Check sheet for the modelled part. Datum: model origin and axes. Units: mm. Face numbers are marked on the shaded views. A direction names the side the tool comes from. Round coordinates to 2 decimals unless told otherwise and drop trailing zeros. Write each loop counter-clockwise with the first axis right and the second up, starting at its lowest first coordinate (ties: lowest second). Pieces come first, ordered by that corner, then holes. Notation, with made-up numbers: M 16.5,60.5 L 57.5,60.5 A22 ccw 57.5,74.5 Z; hole C -37,60.25 d2. An arc over 180 degrees is marked long. Answer in a Markdown table with one row per item.
```python
from build123d import *

# Parameters (mm, degrees)
F0_R     = 11
F1_DEPTH = 1
F2_R     = 9
F3_DEPTH = 7
F4_R     = 11
F5_DEPTH = 8
F6_R     = 0.6
F7_DEPTH = 7
F8_R     = 2.5
F9_DEPTH = 16.001
F10_SIZE = 0.25


with BuildPart() as f1:
    # F0 (on Front) → F1 (new body)
    with BuildSketch(Plane.XZ):
        Circle(F0_R)
    extrude(amount=F1_DEPTH)

    # F2 (on face) → F3 (join)
    with BuildSketch(Plane.XZ.offset(1)):
        Circle(F2_R)
    extrude(amount=F3_DEPTH)

    # F4 (on face) → F5 (join)
    with BuildSketch(Plane.XZ.offset(8)):
        Circle(F4_R)
    extrude(amount=F5_DEPTH)

    # F6 (on face) → F7 (cut, through all)
    with BuildSketch(Plane.XZ.offset(1)):
        with Locations((0, 9)):
            Circle(F6_R)
        with Locations((-1.871205, 8.803328)):
            Circle(F6_R)
        with Locations((-3.66063, 8.221909)):
            Circle(F6_R)
        with Locations((-5.290067, 7.281153)):
            Circle(F6_R)
        with Locations((-6.688303, 6.022175)):
            Circle(F6_R)
        with Locations((-7.794229, 4.5)):
            Circle(F6_R)
        with Locations((-8.559509, 2.781153)):
            Circle(F6_R)
        with Locations((-8.950697, 0.940756)):
            Circle(F6_R)
        with Locations((-8.950697, -0.940756)):
            Circle(F6_R)
        with Locations((-8.559509, -2.781153)):
            Circle(F6_R)
        with Locations((-7.794229, -4.5)):
            Circle(F6_R)
        with Locations((-6.688303, -6.022175)):
            Circle(F6_R)
        with Locations((-5.290067, -7.281153)):
            Circle(F6_R)
        with Locations((-3.66063, -8.221909)):
            Circle(F6_R)
        with Locations((-1.871205, -8.803328)):
            Circle(F6_R)
        with Locations((0, -9)):
            Circle(F6_R)
        with Locations((1.871205, -8.803328)):
            Circle(F6_R)
        with Locations((3.66063, -8.221909)):
            Circle(F6_R)
        with Locations((5.290067, -7.281153)):
            Circle(F6_R)
        with Locations((6.688303, -6.022175)):
            Circle(F6_R)
        with Locations((7.794229, -4.5)):
            Circle(F6_R)
        with Locations((8.559509, -2.781153)):
            Circle(F6_R)
        with Locations((8.950697, -0.940756)):
            Circle(F6_R)
        with Locations((8.950697, 0.940756)):
            Circle(F6_R)
        with Locations((8.559509, 2.781153)):
            Circle(F6_R)
        with Locations((7.794229, 4.5)):
            Circle(F6_R)
        with Locations((6.688303, 6.022175)):
            Circle(F6_R)
        with Locations((5.290067, 7.281153)):
            Circle(F6_R)
        with Locations((3.66063, 8.221909)):
            Circle(F6_R)
        with Locations((1.871205, 8.803328)):
            Circle(F6_R)
    extrude(amount=F7_DEPTH, mode=Mode.SUBTRACT)

    # F8 (on face) → F9 (cut, through all)
    with BuildSketch(Plane.XZ.offset(16)):
        Circle(F8_R)
    extrude(amount=-F9_DEPTH, mode=Mode.SUBTRACT)

    # F10
    f10_edges = [f1.edges().sort_by_distance(p)[0] for p in [
        (11, -12, 0),
        (-11, -8, 0),
        (-11, -16, 0),
        (11, -0.5, 0),
        (-11, 0, 0),
        (-11, -1, 0),
        (-2.5, -16, 0),
        (2.5, -8, 0),
        (-2.5, 0, 0),
    ]]
    chamfer(f10_edges, length=F10_SIZE)


solid = f1.part
```
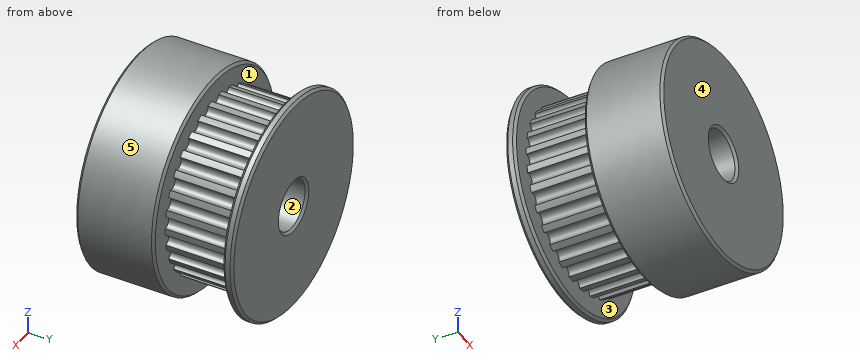
1. Section check B-B, the plane z = 0. Record the cut outline in (x, y), and give its area (3 significant figures).
Found:
| item | result |
|---|---|
| outline | M -11,-15.75 L -10.75,-16 L -2.75,-16 L -2.5,-15.75 L -2.5,-0.25 L -2.75,0 L -10.75,0 L -11,-0.25 L -11,-0.75 L -10.75,-1 L -9,-1 L -9,-8 L -10.75,-8 L -11,-8.25 Z; M 2.5,-15.75 L 2.75,-16 L 10.75,-16 L 11,-15.75 L 11,-8.25 L 10.75,-8 L 9,-8 L 9,-1 L 10.75,-1 L 11,-0.75 L 11,-0.25 L 10.75,0 L 2.75,0 L 2.5,-0.25 Z |
| area | 244 mm2 |
2. Section check C-C, the plane y = -14.25. Record the cut outline in (x, z), and give its area (3 significant figures).
Found:
| item | result |
|---|---|
| outline | C 0,0 d22; hole C 0,0 d5 |
| area | 360 mm2 |
3. Access from +Z, -Z, +X, -X, +Y, -Y to the whole of each face (thin tool, end or side, straight path). Record for the marked faces 1 and 2.
Found:
| item | result |
|---|---|
| face 1 | none |
| face 2 | +Y, -Y |
4. Draft check along Y on the marked faces 3, 4 and 5. Enter one of: +Y half, -Y half, draft (parallel to the pull), parting line (faces both ways), or undercut.
Found:
| item | result |
|---|---|
| face 3 | undercut |
| face 4 | -Y half |
| face 5 | draft |
5. Go/stop test with flat-tipped pins: pin 1 (2 mm diameter, centred on y = -6.5, z = -3.5, fed in from -X); pin 2 (6 mm diameter, centred on x = -8, y = -3, fed in from +Z); pin 3 (1.5 mm diameter, centred on x = 0.5, y = -3.5, fed in from +Z). Record where each tip stops, or that it passes through.
Found:
| item | result |
|---|---|
| pin 1 | stops at x = -8.36 |
| pin 2 | stops at z = 9.21 |
| pin 3 | stops at z = 8.98 |
6. Scan lines: L1, parallel to Z at x = 0, y = -9.75; L2, parallel to Y at x = -9, z = -3.25; L3, parallel to X at y = -2.5, z = -2.75. Record each from-to range of solid material in increasing order.
Found:
| item | result |
|---|---|
| L1 | z = -11 to -2.5, 2.5 to 11 |
| L2 | y = -16 to -8, -1 to 0 |
| L3 | x = -7.96 to 7.96 |
7. Section check A-A, the plane x = 0. Record the cut outline in (y, z).
Found:
| item | result |
|---|---|
| outline | M -16,-10.75 L -15.75,-11 L -8.25,-11 L -8,-10.75 L -8,-8.4 L -1,-8.4 L -1,-10.75 L -0.75,-11 L -0.25,-11 L 0,-10.75 L 0,-2.75 L -0.25,-2.5 L -15.75,-2.5 L -16,-2.75 Z; M -16,2.75 L -15.75,2.5 L -0.25,2.5 L 0,2.75 L 0,10.75 L -0.25,11 L -0.75,11 L -1,10.75 L -1,8.4 L -8,8.4 L -8,10.75 L -8.25,11 L -15.75,11 L -16,10.75 Z |
